CAD build for the part. Positions are in the model's coordinates, mm. A direction names the side the tool comes from. Give positions to 0.01 mm unless a question says otherwise; leave off trailing zeros. Loops run counter-clockwise (first coordinate to the right, second up) from the corner with the lowest first, then second, coordinate; pieces in that order, holes last. Notation, with made-up numbers: M 64.5,68.25 L 70.5,68.25 A26 ccw 70.5,100.25 Z; hole C 69.25,35 d10. An arc over 180 degrees is marked long. One line per question, with ' | ' between items.
```python
from build123d import *

# Parameters (mm, degrees)
SKETCH2_R           = 5.334
SKETCH2_W           = 7.62
SKETCH2_H           = 76.2
BOSS_EXTRUDE1_DEPTH = 2.54
BOSS_EXTRUDE2_START = 24.13
SKETCH3_R           = 5.334
BOSS_EXTRUDE2_DEPTH = 24.13
SKETCH4_W           = 3.175
SKETCH4_H           = 3.175
CUT_EXTRUDE1_DEPTH  = 3.175


with BuildPart() as part:
    # Sketch2 → Boss-Extrude1 (new body)
    with BuildSketch(Plane(origin=(0, 0, 0), x_dir=(1, 0, 0), z_dir=(0, 1, 0))):
        Circle(SKETCH2_R)
        with Locations((0, 38.1)):
            Rectangle(SKETCH2_W, SKETCH2_H)
    extrude(amount=BOSS_EXTRUDE1_DEPTH)

    # Sketch3 → Boss-Extrude2 (add)
    with BuildSketch(Plane.XZ.offset(BOSS_EXTRUDE2_START)):
        with Locations(Location((0, 0, 0), (0, 0, 270))):
            Circle(SKETCH3_R)
    extrude(amount=-BOSS_EXTRUDE2_DEPTH)

    # Sketch4 → Cut-Extrude1 (cut)
    with BuildSketch(Plane.XZ.offset(24.13)):
        with BuildLine():
            Line((-1.5875, -1.5875), (-1.5875, 1.5875))
            Line((-1.5875, 1.5875), (-5.092288263, 1.5875))
            ThreePointArc((-5.092288263, 1.5875), (-5.334, 0), (-5.092288263, -1.5875))
            Line((-5.092288263, -1.5875), (-1.5875, -1.5875))
        make_face()
        Rectangle(SKETCH4_W, SKETCH4_H)
        with BuildLine():
            ThreePointArc((1.5875, 5.092288263), (0, 5.334), (-1.5875, 5.092288263))
            Line((-1.5875, 5.092288263), (-1.5875, 1.5875))
            Line((-1.5875, 1.5875), (1.5875, 1.5875))
            Line((1.5875, 1.5875), (1.5875, 5.092288263))
        make_face()
        with BuildLine():
            Line((5.092288263, 1.5875), (1.5875, 1.5875))
            Line((1.5875, 1.5875), (1.5875, -1.5875))
            Line((1.5875, -1.5875), (5.092288263, -1.5875))
            ThreePointArc((5.092288263, -1.5875), (5.273225843, -0.802898003), (5.334, 0))
            ThreePointArc((5.334, 0), (5.273225843, 0.802898003), (5.092288263, 1.5875))
        make_face()
        with BuildLine():
            Line((1.5875, -1.5875), (-1.5875, -1.5875))
            Line((-1.5875, -1.5875), (-1.5875, -5.092288263))
            ThreePointArc((-1.5875, -5.092288263), (0, -5.334), (1.5875, -5.092288263))
            Line((1.5875, -5.092288263), (1.5875, -1.5875))
        make_face()
    extrude(amount=-CUT_EXTRUDE1_DEPTH, mode=Mode.SUBTRACT)


solid = part.part
```
Item 1: Drill centre lines: line 1 along Y through (x, z) = (-1.5, -56); line 2 along Z through (x, y) = (-0.25, -4); line 3 along Y through (x, z) = (-2.25, -1.5) (3 decimals). Where is each one in solid material? Low to high. Write a range as [from, to].
Conclusion:
line 1: [0, 2.54] | line 2: [-5.33, 5.33] | line 3: [-20.955, 2.54]
Item 2: Saw through at C-C on y = -15. Give the cut face in (x, z), and give its area (3 significant figures).
Conclusion:
outline: C 0,0 d10.67 | area: 89.4 mm²
Item 3: Drop flat-ended pins along their axis: P1, Ø0.8, axis at y = 1, z = -22, coming from the +X side; P2, Ø1.6, axis at x = -3, y = -22, coming from the -Z side; P3, Ø6, axis at x = 1.5, z = -28.5, coming from the -Y side. Give the stop position or say it passes through.
Conclusion:
P1: x = 3.81 | P2: z = -4.86 | P3: y = 0
Item 4: Saw through at A-A on x = 0. Give the cut face in (y, z) (3 decimals), and give its area (3 significant figures).
Conclusion:
outline: M -20.955,-5.334 L 0,-5.334 L 0,-76.2 L 2.54,-76.2 L 2.54,5.334 L -20.955,5.334 Z | area: 431 mm²
Item 5: 3-axis set-ups, long thin cutter, end or side, ignore diameter. For faces 4 (the flat face through (3, -24.13, 3)), 5 (the flat face through (3, -23, -1.588)), 6 (the flat face through (-1.588, -23, 3)), 7 (the flat face through (3.81, 1, -39)), 8 (the flat face through (0, 2.54, -36)): which of +Z, -Z, +X, -X, +Y, -Y reach the whole face in a straight line?
Conclusion:
face 4: +Z, -Z, +X, -X, -Y | face 5: +X, -X, -Y | face 6: +Z, -Z, -Y | face 7: -Z, +X, +Y, -Y | face 8: +Z, -Z, +X, -X, +Y
Item 6: Mould opens along Z. For faces 1 (the flat face through (-3, -23, 1.588)), 2 (the flat face through (0, 1, -76.2)), 3 (the flat face through (-3.81, 1, -39)) say: pulls with the +Z half, pulls with the -Z half, needs draft (parallel to the pull), parting line crosses it, or undercut.
Conclusion:
face 1: undercut | face 2: pulls with the -Z half | face 3: needs draft
Item 7: Saw through at B-B on z = 0. Give the cut face in (x, y) (3 decimals), and give its area (3 significant figures).
Conclusion:
outline: M -5.334,-20.955 L 5.334,-20.955 L 5.334,2.54 L -5.334,2.54 Z | area: 251 mm²
Item 8: Saw through at D-D on z = -56. Give the cut face in (x, y), and give its area (3 significant figures).
Conclusion:
outline: M -3.81,0 L 3.81,0 L 3.81,2.54 L -3.81,2.54 Z | area: 19.4 mm²
